The model under review builds one solid part; all positions refer to its coordinate system, in mm. A direction names the side the tool comes from. Coordinates: 2 decimals unless noted, no trailing zeros. Order: outer loops, then holes, each group sorted by start corner. A loop starts at its lowest first (then second) coordinate and runs counter-clockwise, first axis right, second up. Notation, with made-up numbers: (53.25, 59.25) -> (63.25, 59.25) arc R17 ccw to (63.25, 70.25) -> close; hole circle Ø2 at (72, 86). An arc over 180 degrees is marked (long way). Use one line per item in the form item = value.
from build123d import *

# Parameters (mm, degrees)
F0_W     = 149.225
F0_H     = 3.175
F1_DEPTH = 50.8
F0_H_2   = 146.05
F2_DEPTH = 3.175
F3_W     = 3.175
F3_H     = 152.4
F4_DEPTH = 50.8
F5_W     = 3.175
F5_H     = 152.4
F6_DEPTH = 50.8
F7_R     = 1.7859375
F8_DEPTH = 254


with BuildPart() as f1:
    # F0 (on Top) → F1 (new body)
    with BuildSketch(Plane.XY):
        with Locations((74.6125, 1.5875)):
            Rectangle(F0_W, F0_H)
    extrude(amount=F1_DEPTH)

    # F0 (on Top) → F2 (join)
    with BuildSketch(Plane.XY):
        with Locations((74.6125, 76.2)):
            Rectangle(F0_W, F0_H_2)
    extrude(amount=F2_DEPTH)

    # F3 (on Top) → F4 (join)
    with BuildSketch(Plane.XY):
        with Locations((1.5875, 76.2)):
            Rectangle(F3_W, F3_H)
    extrude(amount=F4_DEPTH)

    # F5 (on Top) → F6 (join)
    with BuildSketch(Plane.XY):
        with Locations((147.6375, 76.2)):
            Rectangle(F5_W, F5_H)
    extrude(amount=F6_DEPTH)

    # F7 (on Right) → F8 (cut)
    with BuildSketch(Plane.YZ):
        with Locations((10.8928065747, 9.9538508803)):
            Circle(F7_R)
        with Locations((22.0790393651, 9.9538508803)):
            Circle(F7_R)
        with Locations((38.5739915073, 9.9538508803)):
            Circle(F7_R)
        with Locations((141.7148411274, 9.9538508803)):
            Circle(F7_R)
        with Locations((128.8222372532, 9.9538508803)):
            Circle(F7_R)
        with Locations((117.8256049752, 9.9538508803)):
            Circle(F7_R)
    extrude(amount=F8_DEPTH, mode=Mode.SUBTRACT)


solid = f1.part
Item 1: Tool access review of faces 4 (the face through (3.175, 77, 31)), 5 (the face through (1.565, 127.405, 8.867)): name each direction out of +Z, -Z, +X, -X, +Y, -Y from which nothing blocks a thin tool from reaching the whole face with its end or side.
Results found:
face_4 = +Z, +Y
face_5 = +X, -X
Item 2: To check wall thickness, follow L1, parallel to X at y = 64.5, z = 14 (3 decimals); L2, parallel to Y at x = 58, z = 25 (3 decimals). State the ranges of each line that lie inside material, in increasing order. Write a range as from..to.
Results found:
L1 = 0..3.175, 146.05..149.225
L2 = 0..3.175
Item 3: Clearance check with flat-ended pins moving along their axes: pin 1 (2 mm diameter, centred on y = 22.08, z = 9.95, fed in from +X); pin 2 (10 mm diameter, centred on x = 104, z = 39.5, fed in from +Y) (3 decimals); pin 3 (2.5 mm diameter, centred on x = 41, z = 1, fed in from +Y) (3 decimals); pin 4 (8 mm diameter, centred on x = 79, y = 115, fed in from +Z) (3 decimals). State where each tip first meets the part, or that it passes through.
Results found:
pin_1 = through
pin_2 = 3.175
pin_3 = 149.225
pin_4 = 3.175
Item 4: We need section A-A (z = 31.5). Write out the cut boundary in (x, y) (3 decimals), plus the area to 3 significant figures.
Results found:
outline = (0, 0) -> (149.225, 0) -> (149.225, 152.4) -> (146.05, 152.4) -> (146.05, 3.175) -> (3.175, 3.175) -> (3.175, 152.4) -> (0, 152.4) -> close
area = 1,420 mm²
Item 5: Draft analysis for pull direction Z (two halves, no side actions). For faces 1 (the face through (149.225, 75, 25)), 2 (the face through (1.57, 21.69, 8.21)), 3 (the face through (2, 77, 50.8)), state which applies: released by +Z, released by -Z, zero draft, split by the parting line, or undercut.
Results found:
face_1 = zero draft
face_2 = undercut
face_3 = released by +Z
Item 6: We need section C-C (x = 139.5). Write out the cut boundary in (y, z) (3 decimals), plus the area to 3 significant figures.
Results found:
outline = (0, 0) -> (149.225, 0) -> (149.225, 3.175) -> (3.175, 3.175) -> (3.175, 50.8) -> (0, 50.8) -> close
area = 625 mm²
Item 7: We need section B-B (y = 137). Write out the cut boundary in (x, z) (3 decimals), plus the area to 3 significant figures.
Results found:
outline = (0, 0) -> (149.225, 0) -> (149.225, 50.8) -> (146.05, 50.8) -> (146.05, 3.175) -> (3.175, 3.175) -> (3.175, 50.8) -> (0, 50.8) -> close
area = 776 mm²
